Design review of the part built by this model. Coordinates are the model's own, in mm. Give positions to 0.01 mm unless a question says otherwise; leave off trailing zeros. Write each loop counter-clockwise with the first axis right and the second up, starting at its lowest first coordinate (ties: lowest second). Pieces come first, ordered by that corner, then holes. Notation, with made-up numbers: (22.25, -11.75) -> (73.25, -11.75) arc R18 cw to (73.25, 5.25) -> close; hole circle Ø6 at (-21, 34.25). An arc over 180 degrees is marked (long way). Put each result on its own line as item: value. Start each with the question number.
Autodesk Inventor part; units mm, degrees
ref_plane "MidSidePlane" through (0, 0, 10) normal (0, 0, 1) x (1, 0, 0)
ref_plane "YZ Plane" through (0, 0, 0) normal (1, 0, 0) x (0, 1, 0)
ref_plane "XZ Plane" through (0, 0, 0) normal (0, 1, 0) x (-1, 0, 0)
sketch "ShaftProfile" plane through (0, 0, 0) normal (0, 0, 1) x (1, 0, 0)
  line L0 (-61, 0) -> (100, 0) construction
  line L1 (-38, 9) -> (77, 9)
  line L2 (77, 9) -> (77, 0)
  line L3 (-38, 0) -> (-38, 9)
  line L4 (-38, 0) -> (77, 0)
  point P0 (0, 0)
  dimension "d1" = 115
  dimension "d2" = 9
  dimension "d4" = 38
revolve "ShaftFeature" add sketch "ShaftProfile" angle 360 about axis through (-38, 0, 0) along (1, 0, 0)
sketch "Sketch2" plane through (-38, 0, 0) normal (-1, 0, 0) x (0, 0, 1)
  circle A0 centre (0, 0) radius 9
hole "ShaftHoleFeature" at (-38, 0, 0) direction (1, 0, 0) diameter 16 end through all
ref_plane "MidSidePlane" through (0, 0, 10) normal (0, 0, 1) x (1, 0, 0)
sketch "CapHoles" plane through (0, 0, 10) normal (0, 0, 1) x (1, 0, 0)
  line L0 (77, -9) -> (77, 9) construction
  line L1 (-38, -9) -> (-38, 9) construction
  line L2 (-56, 0) -> (70, 0) construction
  circle A0 centre (-33.5, 0) radius 1.25
  circle A1 centre (72.5, 0) radius 1.25
  dimension "d24" = 2.5
  dimension "d25" = 4.5
  dimension "d26" = 4.5
extrude "CapHolesFeature" cut sketch "CapHoles" against normal through all
equation "\"d26\" = d25"
properties part number "BackPair1PistonShaft"
Q1. To check wall thickness, follow probe 1 along X at (y, z) = (0, -8.45); probe 2 along Z at (x, y) = (28.5, 0); probe 3 along Y at (x, z) = (44, -0.5). State the ranges of each line that lie inside material, in increasing order. Write a range as from..to.
Q2. Take a section at D-D on y = 5. Give the boundary of the cut face in (x, z) (3 decimals).
Q3. Take a section at C-C on x = 5.5. Give the boundary of the cut face in (y, z), then the cut area to 3 significant figures.
Q4. Take a section at A-A on z = 0. Give the boundary of the cut face in (x, y), then the cut area to 3 significant figures.
Q5. Mouldability with a two-part tool opening along Y and no side actions: class faces 1 (the face through (20.305, -1.172, 8.923)), 2 (the face through (-34.75, 0.05, 8.46)) as +Y half, -Y half, draft (parallel to the pull), parting line (faces both ways), or undercut.
Q6. For pin 1 (4 mm diameter, centred on x = 56.5, y = -6, fed in from -Z); pin 2 (2 mm diameter, centred on y = -5, z = -4, fed in from +X); pin 3 (6 mm diameter, centred on x = -11, z = -5.5, fed in from -Y); pin 4 (1.5 mm diameter, centred on x = -17, z = -6, fed in from -Y), all flat-tipped, find the tip position at first contact; note any pin that passes through.
Q7. Take a section at B-B on y = 0. Give the boundary of the cut face in (x, z), then the cut area to 3 significant figures.
Result:
1. probe 1: x = -38..-34.75, -32.25..71.25, 73.75..77
1. probe 2: z = -9..-8, 8..9
1. probe 3: y = -8.99..-7.98, 7.98..8.99
2. outline: (-38, -7.483) -> (77, -7.483) -> (77, -6.245) -> (-38, -6.245) -> close; (-38, 6.245) -> (77, 6.245) -> (77, 7.483) -> (-38, 7.483) -> close
3. outline: circle Ø18 at (0, 0); hole circle Ø16 at (0, 0)
3. area: 53.4 mm^2
4. outline: (-38, -9) -> (77, -9) -> (77, -8) -> (-38, -8) -> close; (-38, 8) -> (77, 8) -> (77, 9) -> (-38, 9) -> close
4. area: 230 mm^2
5. face 1: parting line
5. face 2: undercut
6. pin 1: stops at z = -8.06
6. pin 2: passes through
6. pin 3: stops at y = -8.65
6. pin 4: stops at y = -7.31
7. outline: (-38, -9) -> (-34.75, -9) -> (-34.75, -8) -> (-38, -8) -> close; (-38, 8) -> (-34.75, 8) -> (-34.75, 9) -> (-38, 9) -> close; (-32.25, -9) -> (71.25, -9) -> (71.25, -8) -> (-32.25, -8) -> close; (-32.25, 8) -> (71.25, 8) -> (71.25, 9) -> (-32.25, 9) -> close; (73.75, -9) -> (77, -9) -> (77, -8) -> (73.75, -8) -> close; (73.75, 8) -> (77, 8) -> (77, 9) -> (73.75, 9) -> close
7. area: 220 mm^2
